Could you check a few things on this drawing? It's one solid part, dimensions in mm from its lowest x, y, z. A direction names the side the tool comes from. Give positions to 0.01 mm unless a question says otherwise; leave off trailing zeros. Loops run counter-clockwise (first coordinate to the right, second up) from the corner with the lowest first, then second, coordinate; pieces in that order, holes last.
Q1. For the marked faces 4, 5 and 6, which set-ups out of +Z, -Z, +X, -X, +Y, -Y let a thin tool reach every point of the face, with its end or its side?
Q2. Suppose I cut it at B-B (x = 12.5). List the corners of the cut face in (y, z) for me.
Q3. I need wall thicknesses on probe 1 along X at (y, z) = (5, 1.25); probe 2 along Z at (x, y) = (1, 4); probe 3 along Y at (x, z) = (5.5, 9.25) (1 decimal). Which ranges of each line are inside material? Lowest first, please.
Q4. I'm going to push flat-ended pins straight in: P1, Ø3, axis at x = 1, y = 4.5, coming from the +Z side; P2, Ø3, axis at x = 10.5, y = 3.5, coming from the -Z side; P3, Ø2, axis at x = 9, z = 2.5, coming from the +Y side; P4, Ø1.4, axis at y = 6, z = 5, coming from the -X side (1 decimal). Where does each tip first touch, or does it pass through?
Q5. Thinking about a two-plate mould opening in Y: for the marked faces 1, 2 and 3, which applies, pulls with the +Y half, pulls with the -Y half, needs draft (parallel to the pull), parting line crosses it, or undercut?
Q6. Suppose I cut it at A-A (x = 2.5). List the corners of the cut face in (y, z) for me.
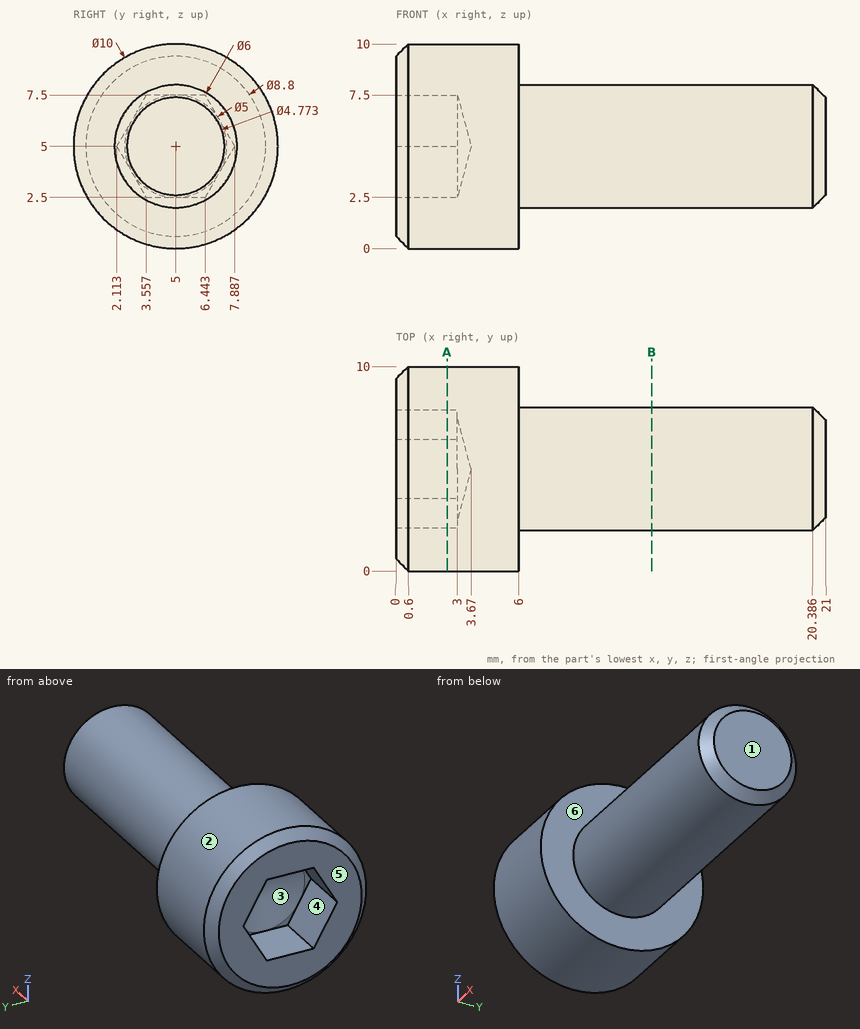
Solutions:
1. face 4: -X
1. face 5: +Z, -Z, -X, +Y, -Y
1. face 6: +X
2. outline: circle Ø6 at (5, 5)
3. probe 1: x = 0 to 6
3. probe 2: z = 0.1 to 2.5, 7.5 to 9.9
3. probe 3: y = 2.4 to 7.6
4. P1: stops at z = 10
4. P2: stops at z = 2
4. P3: stops at y = 7.6
4. P4: stops at x = 3.2
5. face 1: needs draft
5. face 2: parting line crosses it
5. face 3: undercut
6. outline: circle Ø10 at (5, 5); hole (2.11, 5) - (3.56, 2.5) - (6.44, 2.5) - (7.89, 5) - (6.44, 7.5) - (3.56, 7.5) - close
